from build123d import *

# Parameters (mm, degrees)
SKETCH1_W            = 168.91
SKETCH1_H            = 143.51
SKETCH1_W_2          = 133.35
SKETCH1_H_2          = 107.95
BOSS_EXTRUDE1_DEPTH  = 3.175
FILLET1_R            = 6.35
FILLET2_R            = 12.7
SKETCH2_R            = 2.8575
CUT_EXTRUDE1_DEPTH   = 4.175
LPATTERN1_COUNT      = 2
LPATTERN1_PITCH      = 66.548
LPATTERN1_COUNT_DIR2 = 2
LPATTERN1_PITCH_DIR2 = 129.54


with BuildPart() as part:
    # Sketch1 → Boss-Extrude1 (new body)
    with BuildSketch(Plane(origin=(0, 0, 0), x_dir=(1, 0, 0), z_dir=(0, 1, 0))):
        Rectangle(SKETCH1_W, SKETCH1_H)
        Rectangle(SKETCH1_W_2, SKETCH1_H_2, mode=Mode.SUBTRACT)
    extrude(amount=BOSS_EXTRUDE1_DEPTH)

    # Fillet1
    fillet1_edges = [part.edges().sort_by_distance(p)[0] for p in [
        (-84.455, 1.5875, 71.755),
        (-84.455, 1.5875, -71.755),
        (84.455, 1.5875, -71.755),
        (84.455, 1.5875, 71.755),
    ]]
    fillet(fillet1_edges, radius=FILLET1_R)

    # Fillet2
    fillet2_edges = [part.edges().sort_by_distance(p)[0] for p in [
        (-66.675, 1.5875, -53.975),
        (-66.675, 1.5875, 53.975),
        (66.675, 1.5875, 53.975),
        (66.675, 1.5875, -53.975),
    ]]
    fillet(fillet2_edges, radius=FILLET2_R)

    # Sketch2 → Cut-Extrude1 (cut, through all)
    with BuildSketch(Plane(origin=(0, 3.175, 0), x_dir=(1, 0, 0), z_dir=(0, 1, 0))):
        with Locations((-31.6865, 65.405)):
            Circle(SKETCH2_R)
    cut_extrude1 = extrude(amount=-CUT_EXTRUDE1_DEPTH, mode=Mode.SUBTRACT)

    # LPattern1: Cut-Extrude1 2 × 2
    with Locations(*[(i * LPATTERN1_PITCH, 0, j * LPATTERN1_PITCH_DIR2) for i in range(LPATTERN1_COUNT) for j in range(LPATTERN1_COUNT_DIR2) if (i, j) != (0, 0)]):
        add(cut_extrude1, mode=Mode.SUBTRACT)


solid = part.part
Check sheet for the modelled part. Datum: model origin and axes. Units: mm. A direction names the side the tool comes from. Round coordinates to 2 decimals unless told otherwise and drop trailing zeros. Loops run counter-clockwise (first coordinate to the right, second up) from the corner with the lowest first, then second, coordinate; pieces in that order, holes last. Notation, with made-up numbers: M -17.75,-34.75 L 0.25,-34.75 A18 ccw 0.25,-15.75 Z; hole C 25.25,-8.75 d7. An arc over 180 degrees is marked long. One line per question, with ' | ' between items. Start each with the question number.
Item 1: Section check B-B (x = 17). Record the boundary of the cut face in (y, z) (3 decimals), and give its area (3 significant figures).
Item 2: Scan lines: probe 1 along X at (y, z) = (2.3, -37) (3 decimals); probe 2 along Z at (x, y) = (0.5, 2.1) (3 decimals); probe 3 along Z at (x, y) = (56, 1.55) (3 decimals). Record each from-to range of solid material in increasing order.
Item 3: Release check for a two-part mould opening along X. For faces 3 (the face through (-29.047, 1.61, 65.229)), 4 (the face through (-82.64, 1.61, -69.85)), 5 (the face through (-1, 3.175, 63)) record: released by +X, released by -X, zero draft, split by the parting line, or undercut.
Item 4: Section check C-C (y = 2.45). State how many separate pieces and enclosed holes the cut face has, and give its area (3 significant figures).
Item 5: Gauge pin test, flat ends, axial feed: pin 1 Ø6.5 at (x, z) = (34.86, -65.4) entering from -Y; pin 2 Ø5 at (x, z) = (34.86, 64.13) entering from -Y. Record the tip position at first contact, or that the pin passes through.
Item 6: Section check A-A (z = -11). Record the boundary of the cut face in (x, y) (3 decimals).
Item 7: Set-up check for faces 1 (the face through (82.55, 1.61, 69.94)), 2 (the face through (-62.86, 1.61, -50.35)): record each of +Z, -Z, +X, -X, +Y, -Y from which the full face is reachable in a straight line by a thin tool's end or side.
Worked out:
1) outline: M 0,-71.755 L 3.175,-71.755 L 3.175,-53.975 L 0,-53.975 Z; M 0,53.975 L 3.175,53.975 L 3.175,71.755 L 0,71.755 Z | area: 113 mm^2
2) probe 1: -84.455 to -66.675, 66.675 to 84.455 | probe 2: -71.755 to -53.975, 53.975 to 71.755 | probe 3: -71.755 to -53.813, 53.813 to 71.755
3) face 3: undercut | face 4: released by -X | face 5: zero draft
4) separate pieces: 1 | enclosed holes: 5 | area: 9,850 mm^2
5) pin 1: y = 0 | pin 2: through
6) outline: M -84.455,0 L -66.675,0 L -66.675,3.175 L -84.455,3.175 Z; M 66.675,0 L 84.455,0 L 84.455,3.175 L 66.675,3.175 Z
7) face 1: +Z, +X, +Y, -Y | face 2: +Y, -Y
